from build123d import *

# Parameters (mm, degrees)
SKETCH1_W           = 31.8
SKETCH1_H           = 23.5
BOSS_EXTRUDE1_DEPTH = 1.5
SKETCH2_W           = 1.710657602
SKETCH2_H           = 8.486639013
BOSS_EXTRUDE2_DEPTH = 5
SKETCH3_W           = 3.754560192
SKETCH3_H           = 6.242789431
BOSS_EXTRUDE3_DEPTH = 8
SKETCH4_W           = 11.996819547
SKETCH4_H           = 6.420520091
BOSS_EXTRUDE4_DEPTH = 21.5


with BuildPart() as part:
    # Sketch1 → Boss-Extrude1 (new body)
    with BuildSketch(Plane(origin=(0, 0, 0), x_dir=(1, 0, 0), z_dir=(0, 1, 0))):
        with Locations((15.9, -11.75)):
            Rectangle(SKETCH1_W, SKETCH1_H)
    extrude(amount=BOSS_EXTRUDE1_DEPTH)

    # Sketch2 → Boss-Extrude2 (add)
    with BuildSketch(Plane(origin=(0, 1.5, 0), x_dir=(1, 0, 0), z_dir=(0, 1, 0))):
        with Locations((1.148381727, -12.610949144)):
            Rectangle(SKETCH2_W, SKETCH2_H)
    extrude(amount=BOSS_EXTRUDE2_DEPTH)

    # Sketch3 → Boss-Extrude3 (add)
    with BuildSketch(Plane(origin=(0, 1.5, 0), x_dir=(1, 0, 0), z_dir=(0, 1, 0))):
        with Locations((28.985446343, -19.842365371)):
            Rectangle(SKETCH3_W, SKETCH3_H)
    extrude(amount=BOSS_EXTRUDE3_DEPTH)

    # Sketch4 → Boss-Extrude4 (add)
    with BuildSketch(Plane(origin=(0, 1.5, 0), x_dir=(1, 0, 0), z_dir=(0, 1, 0))):
        with Locations((19.310233542, -1.58054006)):
            Rectangle(SKETCH4_W, SKETCH4_H)
    extrude(amount=BOSS_EXTRUDE4_DEPTH)


solid = part.part
Input: part model. Units: mm. Frame: model coordinates. A direction names the side the tool comes from. Coordinates: 2 decimals unless noted, no trailing zeros. Order: outer loops, then holes, each group sorted by start corner. A loop starts at its lowest first (then second) coordinate and runs counter-clockwise, first axis right, second up. Notation, with made-up numbers: M 31,68.5 L 39,68.5 A17 cw 39,97.5 Z; hole C 24.25,74 d1. An arc over 180 degrees is marked long. Answer as CSV lines item,"result".
1. Section B-B (y = 9). Return the cut outline in (x, z), then the cut area to 3 significant figures.
Reported:
outline,"M 13.31,-1.63 L 25.31,-1.63 L 25.31,4.79 L 13.31,4.79 Z; M 27.11,16.72 L 30.86,16.72 L 30.86,22.96 L 27.11,22.96 Z"
area,"100 mm2"
2. Section C-C (x = 22). Return the cut outline in (y, z), then the cut area to 3 significant figures.
Reported:
outline,"M 0,0 L 1.5,0 L 1.5,-1.63 L 23,-1.63 L 23,4.79 L 1.5,4.79 L 1.5,23.5 L 0,23.5 Z"
area,"173 mm2"
3. Section A-A (y = 4.5). Return the cut outline in (x, z).
Reported:
outline,"M 0.29,8.37 L 2,8.37 L 2,16.85 L 0.29,16.85 Z; M 13.31,-1.63 L 25.31,-1.63 L 25.31,4.79 L 13.31,4.79 Z; M 27.11,16.72 L 30.86,16.72 L 30.86,22.96 L 27.11,22.96 Z"
4. Section D-D (z = 3.75). Return the cut outline in (x, y).
Reported:
outline,"M 0,0 L 31.8,0 L 31.8,1.5 L 25.31,1.5 L 25.31,23 L 13.31,23 L 13.31,1.5 L 0,1.5 Z"
5. Access query for faces 1 (the flat face through (25.309, 12, 2)), 2 (the flat face through (16, 1, 0)), 3 (the flat face through (1, 4, 8.368)). Directions: +Z, -Z, +X, -X, +Y, -Y. A direction counts if a zero-diameter tool reaches every point of the face in a straight line with its end or side. Return the directions, or none.
Reported:
face 1,"+Z, -Z, +X, +Y"
face 2,"-Z, +X, -X, -Y"
face 3,"-Z, +X, -X, +Y"
6. First-contact query: P1, Ø12, axis at x = 20.5, y = 15.5, coming from the +Z side; P2, Ø8, axis at y = 16, z = 6, coming from the +X side; P3, Ø12, axis at x = 3.5, z = 13, coming from the +Y side. Flat tips, straight axial feed; report the tip coordinate or a pass-through.
Reported:
P1,"z = 4.79"
P2,"x = 25.31"
P3,"y = 6.5"
7. Material intervals for line 1 (Y direction, x = 30.5, z = 7.75); line 2 (X direction, y = 8, z = 4.25); line 3 (Z direction, x = 25, y = 18), sorted ascending. Write a range as from..to.
Reported:
line 1,"0..1.5"
line 2,"13.31..25.31"
line 3,"-1.63..4.79"
